Autodesk Inventor part; units mm, degrees
ref_plane "YZ Plane" through (0, 0, 0) normal (1, 0, 0) x (0, 1, 0)
ref_plane "XZ Plane" through (0, 0, 0) normal (0, 1, 0) x (-1, 0, 0)
ref_plane "XY Plane" through (0, 0, 0) normal (0, 0, 1) x (1, 0, 0)
sketch "Sketch1" plane through (0, 0, 0) normal (0, 1, 0) x (-1, 0, 0)
  line L0 (37.25, -2.25) -> (24.75, -2.25) construction
  line L1 (24.75, -2.25) -> (24.75, -14.75) construction
  line L2 (24.75, -14.75) -> (37.25, -14.75) construction
  line L3 (37.25, -14.75) -> (37.25, -2.25) construction
  line L4 (56.9183, -8.5) -> (8.3915, -8.5) construction
  line L5 (0, -17) -> (105, -17) construction
  line L6 (0, 0) -> (0, -51) construction
  line L7 (0, -34) -> (105, -34) construction
  line L8 (105, -51) -> (105, 0) construction
  line L9 (31, 19) -> (31, -51) construction
  line L10 (56.8064, -25.5) -> (17, -25.5) construction
  line L11 (24.75, -19.25) -> (24.75, -31.75) construction
  line L12 (37.25, -19.25) -> (24.75, -19.25) construction
  line L13 (37.25, -31.75) -> (37.25, -19.25) construction
  line L14 (24.75, -31.75) -> (37.25, -31.75) construction
  line L15 (24.75, -36.25) -> (24.75, -48.75) construction
  line L16 (37.25, -36.25) -> (24.75, -36.25) construction
  line L17 (37.25, -48.75) -> (37.25, -36.25) construction
  line L18 (24.75, -48.75) -> (37.25, -48.75) construction
  line L19 (56.3008, -42.5) -> (16.5498, -42.5) construction
  arc A0 (53.45, -12) -> (53.45, -22) centre (53.45, -17) ccw
  arc A1 (92, -22) -> (92, -12) centre (92, -17) ccw
  arc A2 (53.45, -29) -> (53.45, -39) centre (53.45, -34) ccw
  arc A3 (92, -39) -> (92, -29) centre (92, -34) ccw
  line L20 (53.45, -12) -> (92, -12)
  line L21 (53.45, -22) -> (92, -22)
  line L22 (53.45, -29) -> (92, -29)
  line L23 (53.45, -39) -> (92, -39)
  arc A4 (16.15, -39) -> (16.15, -29) centre (16.15, -34) ccw
  line L24 (103.5, -49.5) -> (103.5, -1.5) construction
  line L25 (1.5, -1.5) -> (1.5, -49.5) construction
  arc A5 (14, -29) -> (14, -39) centre (14, -34) ccw
  arc A6 (14, -12) -> (14, -22) centre (14, -17) ccw
  line L26 (16.15, -39) -> (14, -39)
  line L27 (14, -29) -> (16.15, -29)
  line L28 (14, -22) -> (16.15, -22)
  line L29 (16.15, -12) -> (14, -12)
  arc A7 (16.15, -22) -> (16.15, -12) centre (16.15, -17) ccw
  arc A8 (96.5, -51) -> (93, -47.5) centre (93, -51) ccw construction
  arc A9 (53.45, -47.5) -> (49.95, -51) centre (53.45, -51) ccw construction
  arc A10 (97.7697, -49.5) -> (93, -46) centre (93, -51) ccw construction
  line L30 (93, -46) -> (53.45, -46) construction
  line L31 (96.5, -51) -> (105, -51) construction
  line L32 (93, -47.5) -> (53.45, -47.5) construction
  line L33 (105, -49.5) -> (97.7697, -49.5) construction
  arc A11 (53.45, -46) -> (48.6803, -49.5) centre (53.45, -51) ccw construction
  arc A12 (48.6803, -1.5) -> (53.45, -5) centre (53.45, 0) ccw construction
  arc A13 (49.95, 0) -> (53.45, -3.5) centre (53.45, 0) ccw construction
  line L34 (93, -3.5) -> (53.45, -3.5) construction
  line L35 (93, -5) -> (53.45, -5) construction
  line L36 (97.7697, -1.5) -> (105, -1.5) construction
  line L37 (105, 0) -> (96.5, 0) construction
  arc A14 (93, -3.5) -> (96.5, 0) centre (93, 0) ccw construction
  arc A15 (93, -5) -> (97.7697, -1.5) centre (93, 0) ccw construction
  arc A16 (16.65, -51) -> (13.15, -47.5) centre (13.15, -51) ccw construction
  arc A17 (12, -47.5) -> (8.5, -51) centre (12, -51) ccw construction
  line L38 (13.15, -46) -> (12, -46) construction
  line L39 (13.15, -47.5) -> (12, -47.5) construction
  arc A18 (12, -46) -> (7.2303, -49.5) centre (12, -51) ccw construction
  arc A19 (17.9197, -49.5) -> (13.15, -46) centre (13.15, -51) ccw construction
  line L40 (48.6803, -49.5) -> (17.9197, -49.5) construction
  line L41 (7.2303, -49.5) -> (0, -49.5) construction
  line L42 (0, -51) -> (8.5, -51) construction
  line L43 (16.65, -51) -> (49.95, -51) construction
  line L44 (13.15, -5) -> (12, -5) construction
  line L45 (13.15, -3.5) -> (12, -3.5) construction
  arc A20 (8.5, 0) -> (12, -3.5) centre (12, 0) ccw construction
  arc A21 (13.15, -3.5) -> (16.65, 0) centre (13.15, 0) ccw construction
  arc A22 (7.2303, -1.5) -> (12, -5) centre (12, 0) ccw construction
  arc A23 (13.15, -5) -> (17.9197, -1.5) centre (13.15, 0) ccw construction
  line L46 (49.95, 0) -> (16.65, 0) construction
  line L47 (8.5, 0) -> (0, 0) construction
  line L48 (0, -1.5) -> (7.2303, -1.5) construction
  line L49 (17.9197, -1.5) -> (48.6803, -1.5) construction
  arc A24 (38.75, -4.25) -> (35.25, -0.75) centre (35.25, -4.25) ccw
  arc A25 (26.75, -0.75) -> (23.25, -4.25) centre (26.75, -4.25) ccw
  arc A26 (35.25, -50.25) -> (38.75, -46.75) centre (35.25, -46.75) ccw
  arc A27 (23.25, -46.75) -> (26.75, -50.25) centre (26.75, -46.75) ccw
  line L50 (38.75, -4.25) -> (38.75, -46.75)
  line L51 (35.25, -0.75) -> (26.75, -0.75)
  line L52 (23.25, -4.25) -> (23.25, -46.75)
  line L53 (26.75, -50.25) -> (35.25, -50.25)
  line L54 (119, -53) -> (119, -56)
  line L55 (-77, -56) -> (-77, -53)
  line L56 (119, 2) -> (119, 5)
  line L57 (-77, 5) -> (-77, 2)
  line L58 (51, -56) -> (51, -53)
  line L59 (11, -56) -> (11, -53)
  line L60 (71, -56) -> (71, -53)
  line L61 (94, -53) -> (94, -56)
  line L62 (-9, -53) -> (-9, -56)
  line L63 (-59, -56) -> (-59, -53)
  line L64 (94, 2) -> (94, 5)
  line L65 (71, 2) -> (71, 5)
  line L66 (51, 2) -> (51, 5)
  line L67 (11, 2) -> (11, 5)
  line L68 (-9, 2) -> (-9, 5)
  line L69 (-59, 2) -> (-59, 5)
  line L70 (122, -56) -> (122, 5)
  line L71 (-80, 5) -> (-80, -56)
  line L72 (122, -56) -> (122, -59)
  line L73 (122, -59) -> (-80, -59)
  line L74 (-80, -59) -> (-80, -56)
  line L75 (122, 5) -> (122, 8)
  line L76 (122, 8) -> (-80, 8)
  line L77 (-80, 8) -> (-80, 5)
  line L78 (119, -56) -> (94, -56)
  line L79 (71, -56) -> (51, -56)
  line L80 (11, -56) -> (-9, -56)
  line L81 (-59, -56) -> (-77, -56)
  line L82 (-59, -53) -> (-77, -53)
  line L83 (-9, -53) -> (11, -53)
  line L84 (51, -53) -> (71, -53)
  line L85 (94, -53) -> (119, -53)
  line L86 (119, 5) -> (94, 5)
  line L87 (119, 2) -> (94, 2)
  line L88 (71, 2) -> (51, 2)
  line L89 (71, 5) -> (51, 5)
  line L90 (11, 2) -> (-9, 2)
  line L91 (11, 5) -> (-9, 5)
  line L92 (-59, 2) -> (-77, 2)
  line L93 (-59, 5) -> (-77, 5)
  line L94 (-24, -53) -> (-39, -53)
  line L95 (-39, -53) -> (-39, -56)
  line L96 (-39, -56) -> (-24, -56)
  line L97 (-24, -56) -> (-24, -53)
  line L98 (-24, 5) -> (-39, 5)
  line L99 (-39, 5) -> (-39, 2)
  line L100 (-39, 2) -> (-24, 2)
  line L101 (-24, 2) -> (-24, 5)
  line L102 (-74, -8) -> (-77, -8)
  line L103 (-77, -8) -> (-77, -18)
  line L104 (-77, -18) -> (-74, -18)
  line L105 (-74, -18) -> (-74, -8)
  line L106 (-74, -33) -> (-77, -33)
  line L107 (-77, -33) -> (-77, -43)
  line L108 (-77, -43) -> (-74, -43)
  line L109 (-74, -43) -> (-74, -33)
  line L110 (119, -8) -> (116, -8)
  line L111 (116, -8) -> (116, -18)
  line L112 (116, -18) -> (119, -18)
  line L113 (119, -18) -> (119, -8)
  line L114 (119, -33) -> (116, -33)
  line L115 (116, -33) -> (116, -43)
  line L116 (116, -43) -> (119, -43)
  line L117 (119, -43) -> (119, -33)
  line L118 (-74, 2) -> (-67, 2) construction
  line L119 (-74, -18) -> (-76.75, -18) construction
  line L120 (-76.75, -33) -> (-74, -33) construction
  circle A28 centre (-48.5, -42.5) radius 2.5
  circle A29 centre (-48.5, -25.5) radius 2.5
  circle A30 centre (-48.5, -8.5) radius 2.5
  point P0 (31, -8.5)
  point P1 (31, -42.5)
  point P2 (31, -25.5)
  point P3 (-74, -53)
  point P4 (-74, -53)
  point P5 (-74, -53)
  point P6 (-74, -53)
  dimension "d0" = 12.5
  dimension "d1" = 12.5
  dimension "d2" = 17
  dimension "d3" = 31
  dimension "d4" = 105
  dimension "d5" = 17
  dimension "d6" = 17
  dimension "d7" = 10
  dimension "d8" = 1.5
  dimension "d9" = 1.5
  dimension "d10" = 5
  dimension "d11" = 1.5
  dimension "d12" = 1.5
  dimension "d13" = 1.5
  dimension "d14" = 17
  dimension "d15" = 17
  dimension "d16" = 12
  dimension "d17" = 13
  dimension "d19" = 11.6
  dimension "d20" = 8.6
  dimension "d21" = 12
  dimension "d28" = 2
  dimension "d29" = 2
  dimension "d30" = 7
  dimension "d31" = 2
  dimension "d32" = 2
  dimension "d38" = 40
  dimension "d39" = 20
  dimension "d40" = 23
  dimension "d42" = 20
  dimension "d46" = 202
  dimension "d55" = 3
  dimension "d56" = 3
  dimension "d60" = 18
  dimension "d61" = 15
  dimension "d62" = 15
  dimension "d63" = 20
  dimension "d64" = 14
  dimension "d65" = 22.45
  dimension "d66" = 10.5
  dimension "d67" = 2
  dimension "d73" = 25
  dimension "d74" = 3
  dimension "d78" = 3
  dimension "d79" = 3
  dimension "d80" = 15
  dimension "d81" = 10
  dimension "d92" = 2.75
  dimension "d100" = 17
  dimension "d105" = 20
  dimension "d107" = 15
  dimension "d109" = 5
  dimension "d110" = 31.5
  dimension "d111" = 16.5
  dimension "d112" = 17
extrude "Extrusion2" add sketch "Sketch1" along normal blind 3
properties part number "Top_plate2"
Input: part model. Units: mm. Frame: model coordinates. A direction names the side the tool comes from. Coordinates: 2 decimals unless noted, no trailing zeros. Loops run counter-clockwise (first coordinate to the right, second up) from the corner with the lowest first, then second, coordinate; pieces in that order, holes last. Notation, with made-up numbers: (22.25, 27) -> (72.25, 27) arc R38 cw to (72.25, 65) -> close; hole circle Ø8 at (36.5, 73). An arc over 180 degrees is marked (long way). Write item = value, one per line. Start each with the question number.
Item 1: Mould query, pull axis X, two halves, no side actions, for faces 1 (the face through (-48.45, 1.48, -17.11)), 2 (the face through (-20, 3, -25)). Classes: pulls with the +X half, pulls with the -X half, needs draft (parallel to the pull), parting line crosses it, or undercut.
Item 2: Cut plane C-C, the plane x = 48. Return loops of the section in (y, z), plus the area to 3 significant figures.
Item 3: Reachability of faces 3 (the face through (-20, 0, -25)), 4 (the face through (-37.7, 1.48, -1.75)) from +Z, -Z, +X, -X, +Y, -Y: full face, straight path, thin tool, end or side. Return the list, or none.
Item 4: Material intervals for line 1 (Z direction, x = -101, y = 2.4); line 2 (Z direction, x = 48.5, y = 2.3); line 3 (Z direction, x = -70, y = 2.7), sorted ascending.
Item 5: Cut plane A-A, the plane x = 4. Return loops of the section in (y, z), plus the area to 3 significant figures.
Item 6: Cut plane D-D, the plane x = -82. Return loops of the section in (y, z).
Item 7: Cut plane B-B, the plane z = -31. Return loops of the section in (x, y), plus the area to 3 significant figures.
Item 8: First-contact query: P1, Ø4, axis at x = 48.5, z = -8.5, coming from the +Y side. Flat tip, straight axial feed; report the tip coordinate or a pass-through.
Ans:
q1.face_1 = undercut
q1.face_2 = needs draft
q2.outline = (0, -59) -> (3, -59) -> (3, -44.95) -> (0, -44.95) -> close; (0, -40.05) -> (3, -40.05) -> (3, -27.95) -> (0, -27.95) -> close; (0, -23.05) -> (3, -23.05) -> (3, -10.95) -> (0, -10.95) -> close; (0, -6.05) -> (3, -6.05) -> (3, 8) -> (0, 8) -> close
q2.area = 157 mm²
q3.face_3 = +Z, -Z, +X, -X, -Y
q3.face_4 = +Y, -Y
q4.line_1 = -59 to -56, -53 to 2, 5 to 8
q4.line_2 = -59 to -45, -40 to -28, -23 to -11, -6 to 8
q4.line_3 = -59 to -56, -53 to -39, -29 to -22, -12 to 2, 5 to 8
q5.outline = (0, -59) -> (3, -59) -> (3, -56) -> (0, -56) -> close; (0, -53) -> (3, -53) -> (3, 2) -> (0, 2) -> close; (0, 5) -> (3, 5) -> (3, 8) -> (0, 8) -> close
q5.area = 183 mm²
q6.outline = (0, -59) -> (3, -59) -> (3, -39) -> (0, -39) -> close; (0, -29) -> (3, -29) -> (3, -22) -> (0, -22) -> close; (0, -12) -> (3, -12) -> (3, 8) -> (0, 8) -> close
q7.outline = (-122, 0) -> (-96, 0) -> (-96, 3) -> (-122, 3) -> close; (-49.45, 0) -> (-38.75, 0) -> (-38.75, 3) -> (-49.45, 3) -> close; (-23.25, 0) -> (-20.15, 0) -> (-20.15, 3) -> (-23.25, 3) -> close; (-10, 0) -> (80, 0) -> (80, 3) -> (-10, 3) -> close
q7.area = 389 mm²
q8.P1 = through
